```python
from build123d import *
from OCP.BRepFilletAPI import BRepFilletAPI_MakeChamfer

# Parameters (mm, degrees)
BOSS_EXTRUDE1_DEPTH       = 5
FILLET1_R                 = 4
SKETCH2_R                 = 8
BOSS_EXTRUDE2_DEPTH       = 1
SKETCH3_R                 = 8
BOSS_EXTRUDE3_DEPTH       = 1
SKETCH4_R                 = 6
CUT_EXTRUDE1_DEPTH        = 44.235891121
CUT_EXTRUDE2_DEPTH        = 2
CHAMFER1_SIZE             = 1
CHAMFER1_SIZE2            = 1.732050808
CHAMFER1_OF_MIRROR3_SIZE  = 1
CHAMFER1_OF_MIRROR3_SIZE2 = 1.732050808
SKETCH6_R                 = 1.5
CUT_EXTRUDE3_DEPTH        = 42.968348563
CUT_EXTRUDE3_DEPTH_BACK   = 42.968348563


with BuildPart() as part:
    # Sketch1 → Boss-Extrude1 (new, symmetric)
    with BuildSketch(Plane(origin=(0, 0, 0), x_dir=(1, 0, 0), z_dir=(0, 1, 0))):
        with BuildLine():
            Line((-10, 30.489995997), (-10, -2.679491924))
            Line((-10, -2.679491924), (-25.114071484, -6.729295173))
            ThreePointArc((-25.114071484, -6.729295173), (0, -26), (25.114071484, -6.729295173))
            Line((25.114071484, -6.729295173), (10, -2.679491924))
            Line((10, -2.679491924), (10, 30.489995997))
            ThreePointArc((10, 30.489995997), (0, 34), (-10, 30.489995997))
        make_face()
    extrude(amount=BOSS_EXTRUDE1_DEPTH, both=True)

    # Fillet1
    fillet1_edges = [part.edges().sort_by_distance(p)[0] for p in [
        (10, 0, -30.489995997),
        (10, 0, 2.679491924),
        (25.114071484, 0, 6.729295173),
        (-25.114071484, 0, 6.729295173),
        (-10, 0, 2.679491924),
        (-10, 0, -30.489995997),
    ]]
    fillet(fillet1_edges, radius=FILLET1_R)

    # Sketch2 → Boss-Extrude2 (add)
    with BuildSketch(Plane.XZ.offset(5)):
        with Locations(Location((0, 0, 0), (0, 0, 90))):
            Circle(SKETCH2_R)
    extrude(amount=BOSS_EXTRUDE2_DEPTH)

    # Sketch3 → Boss-Extrude3 (add)
    with BuildSketch(Plane(origin=(0, 5, 0), x_dir=(1, 0, 0), z_dir=(0, 1, 0))):
        with Locations(Location((0, 18, 0), (0, 0, 270))):
            Circle(SKETCH3_R)
    extrude(amount=BOSS_EXTRUDE3_DEPTH)

    # Sketch4 → Cut-Extrude1 (cut, through all)
    with BuildSketch(Plane.XZ.offset(6)):
        with Locations(Location((0, 0, 0), (0, 0, 270))):
            Circle(SKETCH4_R)
        with Locations(Location((0, -18, 0), (0, 0, 270))):
            Circle(SKETCH4_R)
    extrude(amount=-CUT_EXTRUDE1_DEPTH, mode=Mode.SUBTRACT)

    # Sketch5 → Cut-Extrude2 (cut)
    with BuildSketch(Plane(origin=(0, 5, 0), x_dir=(1, 0, 0), z_dir=(0, 1, 0))):
        with BuildLine():
            Line((12.188266684, -6.371664756), (20.119713435, -8.496889508))
            ThreePointArc((20.119713435, -8.496889508), (20.768948696, -9.043962883), (20.763662316, -9.892943304))
            ThreePointArc((20.763662316, -9.892943304), (0, -23), (-20.763662316, -9.892943304))
            ThreePointArc((-20.763662316, -9.892943304), (-20.768948696, -9.043962883), (-20.119713435, -8.496889508))
            Line((-20.119713435, -8.496889508), (-12.188266684, -6.371664756))
            ThreePointArc((-12.188266684, -6.371664756), (-11.342355786, -6.086056673), (-10.539679728, -5.695098402))
            ThreePointArc((-10.539679728, -5.695098402), (-9.810114884, -5.592432974), (-9.208235905, -6.017340901))
            ThreePointArc((-9.208235905, -6.017340901), (0, -11), (9.208235905, -6.017340901))
            ThreePointArc((9.208235905, -6.017340901), (9.810114884, -5.592432974), (10.539679728, -5.695098402))
            ThreePointArc((10.539679728, -5.695098402), (11.342355786, -6.086056673), (12.188266684, -6.371664756))
        make_face()
    cut_extrude2 = extrude(amount=-CUT_EXTRUDE2_DEPTH, mode=Mode.SUBTRACT)

    # Chamfer1: one chamfer whose edges measure the first distance from different faces: ONE call of the kernel's chamfer builder (chamfer() names one face for all edges)
    chamfer1_edges_1 = [part.edges().sort_by_distance(p)[0] for p in [
        (9.810114884, 5, 5.592432974),
    ]]
    chamfer1_side_1 = [part.faces().sort_by_distance(p)[0] for p in [
        (9.810114884, 4, 5.592432974),
    ]]
    chamfer1_edges_2 = [part.edges().sort_by_distance(p)[0] for p in [
        (0, 5, 11),
    ]]
    chamfer1_side_2 = [part.faces().sort_by_distance(p)[0] for p in [
        (0, 4, 11),
    ]]
    chamfer1_edges_3 = [part.edges().sort_by_distance(p)[0] for p in [
        (-9.810114884, 5, 5.592432974),
    ]]
    chamfer1_side_3 = [part.faces().sort_by_distance(p)[0] for p in [
        (-9.810114884, 4, 5.592432974),
    ]]
    chamfer1_edges_4 = [part.edges().sort_by_distance(p)[0] for p in [
        (-11.342355786, 5, 6.086056673),
    ]]
    chamfer1_side_4 = [part.faces().sort_by_distance(p)[0] for p in [
        (-11.342355786, 4, 6.086056673),
    ]]
    chamfer1_edges_5 = [part.edges().sort_by_distance(p)[0] for p in [
        (-16.153990059, 5, 7.434277132),
    ]]
    chamfer1_side_5 = [part.faces().sort_by_distance(p)[0] for p in [
        (-16.153990059, 4, 7.434277132),
    ]]
    chamfer1_edges_6 = [part.edges().sort_by_distance(p)[0] for p in [
        (-20.768948696, 5, 9.043962883),
    ]]
    chamfer1_side_6 = [part.faces().sort_by_distance(p)[0] for p in [
        (-20.768948696, 4, 9.043962883),
    ]]
    chamfer1_edges_7 = [part.edges().sort_by_distance(p)[0] for p in [
        (0, 5, 23),
    ]]
    chamfer1_side_7 = [part.faces().sort_by_distance(p)[0] for p in [
        (0, 4, 23),
    ]]
    chamfer1_edges_8 = [part.edges().sort_by_distance(p)[0] for p in [
        (20.768948696, 5, 9.043962883),
    ]]
    chamfer1_side_8 = [part.faces().sort_by_distance(p)[0] for p in [
        (20.768948696, 4, 9.043962883),
    ]]
    chamfer1_edges_9 = [part.edges().sort_by_distance(p)[0] for p in [
        (16.153990059, 5, 7.434277132),
    ]]
    chamfer1_side_9 = [part.faces().sort_by_distance(p)[0] for p in [
        (16.153990059, 4, 7.434277132),
    ]]
    chamfer1_edges_10 = [part.edges().sort_by_distance(p)[0] for p in [
        (11.342355786, 5, 6.086056673),
    ]]
    chamfer1_side_10 = [part.faces().sort_by_distance(p)[0] for p in [
        (11.342355786, 4, 6.086056673),
    ]]
    chamfer1 = BRepFilletAPI_MakeChamfer(part.part.solid().wrapped)
    for e in chamfer1_edges_1:
        chamfer1.Add(CHAMFER1_SIZE, CHAMFER1_SIZE2, e.wrapped, chamfer1_side_1[0].wrapped)  # the first distance lies on this face
    for e in chamfer1_edges_2:
        chamfer1.Add(CHAMFER1_SIZE, CHAMFER1_SIZE2, e.wrapped, chamfer1_side_2[0].wrapped)  # the first distance lies on this face
    for e in chamfer1_edges_3:
        chamfer1.Add(CHAMFER1_SIZE, CHAMFER1_SIZE2, e.wrapped, chamfer1_side_3[0].wrapped)  # the first distance lies on this face
    for e in chamfer1_edges_4:
        chamfer1.Add(CHAMFER1_SIZE, CHAMFER1_SIZE2, e.wrapped, chamfer1_side_4[0].wrapped)  # the first distance lies on this face
    for e in chamfer1_edges_5:
        chamfer1.Add(CHAMFER1_SIZE, CHAMFER1_SIZE2, e.wrapped, chamfer1_side_5[0].wrapped)  # the first distance lies on this face
    for e in chamfer1_edges_6:
        chamfer1.Add(CHAMFER1_SIZE, CHAMFER1_SIZE2, e.wrapped, chamfer1_side_6[0].wrapped)  # the first distance lies on this face
    for e in chamfer1_edges_7:
        chamfer1.Add(CHAMFER1_SIZE, CHAMFER1_SIZE2, e.wrapped, chamfer1_side_7[0].wrapped)  # the first distance lies on this face
    for e in chamfer1_edges_8:
        chamfer1.Add(CHAMFER1_SIZE, CHAMFER1_SIZE2, e.wrapped, chamfer1_side_8[0].wrapped)  # the first distance lies on this face
    for e in chamfer1_edges_9:
        chamfer1.Add(CHAMFER1_SIZE, CHAMFER1_SIZE2, e.wrapped, chamfer1_side_9[0].wrapped)  # the first distance lies on this face
    for e in chamfer1_edges_10:
        chamfer1.Add(CHAMFER1_SIZE, CHAMFER1_SIZE2, e.wrapped, chamfer1_side_10[0].wrapped)  # the first distance lies on this face
    add(Compound.cast(chamfer1.Shape()), mode=Mode.REPLACE)

    # Mirror3: Cut-Extrude2 across plane
    add(cut_extrude2.mirror(Plane.ZX), mode=Mode.SUBTRACT)

    # Chamfer1 of Mirror3: one chamfer whose edges measure the first distance from different faces: ONE call of the kernel's chamfer builder (chamfer() names one face for all edges)
    chamfer1_of_mirror3_edges_1 = [part.edges().sort_by_distance(p)[0] for p in [
        (9.810114884, -5, 5.592432974),
    ]]
    chamfer1_of_mirror3_side_1 = [part.faces().sort_by_distance(p)[0] for p in [
        (9.810114884, -4, 5.592432974),
    ]]
    chamfer1_of_mirror3_edges_2 = [part.edges().sort_by_distance(p)[0] for p in [
        (0, -5, 11),
    ]]
    chamfer1_of_mirror3_side_2 = [part.faces().sort_by_distance(p)[0] for p in [
        (0, -4, 11),
    ]]
    chamfer1_of_mirror3_edges_3 = [part.edges().sort_by_distance(p)[0] for p in [
        (-9.810114884, -5, 5.592432974),
    ]]
    chamfer1_of_mirror3_side_3 = [part.faces().sort_by_distance(p)[0] for p in [
        (-9.810114884, -4, 5.592432974),
    ]]
    chamfer1_of_mirror3_edges_4 = [part.edges().sort_by_distance(p)[0] for p in [
        (-11.342355786, -5, 6.086056673),
    ]]
    chamfer1_of_mirror3_side_4 = [part.faces().sort_by_distance(p)[0] for p in [
        (-11.342355786, -4, 6.086056673),
    ]]
    chamfer1_of_mirror3_edges_5 = [part.edges().sort_by_distance(p)[0] for p in [
        (-16.153990059, -5, 7.434277132),
    ]]
    chamfer1_of_mirror3_side_5 = [part.faces().sort_by_distance(p)[0] for p in [
        (-16.153990059, -4, 7.434277132),
    ]]
    chamfer1_of_mirror3_edges_6 = [part.edges().sort_by_distance(p)[0] for p in [
        (-20.768948696, -5, 9.043962883),
    ]]
    chamfer1_of_mirror3_side_6 = [part.faces().sort_by_distance(p)[0] for p in [
        (-20.768948696, -4, 9.043962883),
    ]]
    chamfer1_of_mirror3_edges_7 = [part.edges().sort_by_distance(p)[0] for p in [
        (0, -5, 23),
    ]]
    chamfer1_of_mirror3_side_7 = [part.faces().sort_by_distance(p)[0] for p in [
        (0, -4, 23),
    ]]
    chamfer1_of_mirror3_edges_8 = [part.edges().sort_by_distance(p)[0] for p in [
        (20.768948696, -5, 9.043962883),
    ]]
    chamfer1_of_mirror3_side_8 = [part.faces().sort_by_distance(p)[0] for p in [
        (20.768948696, -4, 9.043962883),
    ]]
    chamfer1_of_mirror3_edges_9 = [part.edges().sort_by_distance(p)[0] for p in [
        (16.153990059, -5, 7.434277132),
    ]]
    chamfer1_of_mirror3_side_9 = [part.faces().sort_by_distance(p)[0] for p in [
        (16.153990059, -4, 7.434277132),
    ]]
    chamfer1_of_mirror3_edges_10 = [part.edges().sort_by_distance(p)[0] for p in [
        (11.342355786, -5, 6.086056673),
    ]]
    chamfer1_of_mirror3_side_10 = [part.faces().sort_by_distance(p)[0] for p in [
        (11.342355786, -4, 6.086056673),
    ]]
    chamfer1_of_mirror3 = BRepFilletAPI_MakeChamfer(part.part.solid().wrapped)
    for e in chamfer1_of_mirror3_edges_1:
        chamfer1_of_mirror3.Add(CHAMFER1_OF_MIRROR3_SIZE, CHAMFER1_OF_MIRROR3_SIZE2, e.wrapped, chamfer1_of_mirror3_side_1[0].wrapped)  # the first distance lies on this face
    for e in chamfer1_of_mirror3_edges_2:
        chamfer1_of_mirror3.Add(CHAMFER1_OF_MIRROR3_SIZE, CHAMFER1_OF_MIRROR3_SIZE2, e.wrapped, chamfer1_of_mirror3_side_2[0].wrapped)  # the first distance lies on this face
    for e in chamfer1_of_mirror3_edges_3:
        chamfer1_of_mirror3.Add(CHAMFER1_OF_MIRROR3_SIZE, CHAMFER1_OF_MIRROR3_SIZE2, e.wrapped, chamfer1_of_mirror3_side_3[0].wrapped)  # the first distance lies on this face
    for e in chamfer1_of_mirror3_edges_4:
        chamfer1_of_mirror3.Add(CHAMFER1_OF_MIRROR3_SIZE, CHAMFER1_OF_MIRROR3_SIZE2, e.wrapped, chamfer1_of_mirror3_side_4[0].wrapped)  # the first distance lies on this face
    for e in chamfer1_of_mirror3_edges_5:
        chamfer1_of_mirror3.Add(CHAMFER1_OF_MIRROR3_SIZE, CHAMFER1_OF_MIRROR3_SIZE2, e.wrapped, chamfer1_of_mirror3_side_5[0].wrapped)  # the first distance lies on this face
    for e in chamfer1_of_mirror3_edges_6:
        chamfer1_of_mirror3.Add(CHAMFER1_OF_MIRROR3_SIZE, CHAMFER1_OF_MIRROR3_SIZE2, e.wrapped, chamfer1_of_mirror3_side_6[0].wrapped)  # the first distance lies on this face
    for e in chamfer1_of_mirror3_edges_7:
        chamfer1_of_mirror3.Add(CHAMFER1_OF_MIRROR3_SIZE, CHAMFER1_OF_MIRROR3_SIZE2, e.wrapped, chamfer1_of_mirror3_side_7[0].wrapped)  # the first distance lies on this face
    for e in chamfer1_of_mirror3_edges_8:
        chamfer1_of_mirror3.Add(CHAMFER1_OF_MIRROR3_SIZE, CHAMFER1_OF_MIRROR3_SIZE2, e.wrapped, chamfer1_of_mirror3_side_8[0].wrapped)  # the first distance lies on this face
    for e in chamfer1_of_mirror3_edges_9:
        chamfer1_of_mirror3.Add(CHAMFER1_OF_MIRROR3_SIZE, CHAMFER1_OF_MIRROR3_SIZE2, e.wrapped, chamfer1_of_mirror3_side_9[0].wrapped)  # the first distance lies on this face
    for e in chamfer1_of_mirror3_edges_10:
        chamfer1_of_mirror3.Add(CHAMFER1_OF_MIRROR3_SIZE, CHAMFER1_OF_MIRROR3_SIZE2, e.wrapped, chamfer1_of_mirror3_side_10[0].wrapped)  # the first distance lies on this face
    add(Compound.cast(chamfer1_of_mirror3.Shape()), mode=Mode.REPLACE)

    # Sketch6 → Cut-Extrude3 (cut, two sides)
    with BuildSketch(Plane(origin=(0, 0, 0), x_dir=(0, 0, -1), z_dir=(1, 0, 0))) as cut_extrude3_sk:
        Circle(SKETCH6_R)
        with Locations((18, 0)):
            Circle(SKETCH6_R)
    extrude(amount=CUT_EXTRUDE3_DEPTH, mode=Mode.SUBTRACT)
    extrude(cut_extrude3_sk.sketch, amount=-CUT_EXTRUDE3_DEPTH_BACK, mode=Mode.SUBTRACT)


solid = part.part
```
Verification items for the finished model (mm, model axes). A direction names the side the tool comes from. Give positions to 0.01 mm unless a question says otherwise; leave off trailing zeros. Order: outer loops, then holes, each group sorted by start corner. A loop starts at its lowest first (then second) coordinate and runs counter-clockwise, first axis right, second up. Notation, with made-up numbers: M 44.5,-11.75 L 80.5,-11.75 A37 ccw 80.5,25.25 Z; hole C 67,44 d7. An arc over 180 degrees is marked long. Answer in a Markdown table with one row per item. Add a question column.
Item 1: Section check C-C, the plane x = 0. State how many separate pieces and enclosed holes the cut face has, and give its area (3 significant figures).
Item 2: Scan lines: probe 1 along X at (y, z) = (-1.75, -18); probe 2 along Z at (x, y) = (8, 0); probe 3 along Z at (x, y) = (7.95, 0). Record each from-to range of solid material in increasing order. Write a range as from..to.
Item 3: Mould release check, pull along Z, two halves, no side actions. Record for faces 4 (the flat face through (16.986, 0.07, 4.551)), 5 (the cylindrical face through (23.47, 0.07, 7.74)), 6 (the flat face through (0, -3, 14)): released by +Z, released by -Z, zero draft, split by the parting line, or undercut.
Item 4: Section check A-A, the plane y = 0. Enter the section's corners in (x, z).
Item 5: Section check B-B, the plane z = -18. Enter the section's corners in (x, y), and give its area (3 significant figures).
Item 6: Tool access check on faces 1 (the flat face through (16.33, -4.51, 6.57)), 2 (the flat face through (-16.21, 3.51, 7.45)), 3 (the flat face through (-10, 0, -15)). Record the directions out of +Z, -Z, +X, -X, +Y, -Y that give a thin tool (end or side, any length) a straight path to the whole face; none if there is none.
Item 7: Gauge pin test, flat ends, axial feed: pin 1 (10 mm diameter, centred on x = 7.5, z = -5.5, fed in from +Y); pin 2 (3 mm diameter, centred on x = -10, y = 4, fed in from -Z); pin 3 (5 mm diameter, centred on y = 0, z = 0, fed in from +X). Record the tip position at first contact, or that the pin passes through.
Filled sheet:
| question | item | result |
|---|---|---|
| 1 | separate pieces | 3 |
| 1 | enclosed holes | 0 |
| 1 | area | 317 mm^2 |
| 2 | probe 1 | x = -10..-6, 6..10 |
| 2 | probe 2 | z = -31.86..-19.5, -16.5..-1.5, 1.5..24.74 |
| 2 | probe 3 | z = -31.89..-19.5, -16.5..-1.5, 1.5..24.75 |
| 3 | face 4 | released by -Z |
| 3 | face 5 | split by the parting line |
| 3 | face 6 | undercut |
| 4 | outline | M -23.47,11.18 A4 ccw -20.9,5.6 L -12.96,3.47 A4 cw -10.47,1.5 L -5.81,1.5 A6 cw 5.81,1.5 L 10.47,1.5 A4 cw 12.96,3.47 L 20.9,5.6 A4 ccw 23.47,11.18 A26 ccw Z; M -10,-28.39 A4 ccw -8,-31.86 A16 ccw 8,-31.86 A4 ccw 10,-28.39 L 10,-19.5 L 5.81,-19.5 A6 cw -5.81,-19.5 L -10,-19.5 Z; M -10,-16.5 L -5.81,-16.5 A6 cw 5.81,-16.5 L 10,-16.5 L 10,-1.5 L 5.81,-1.5 A6 cw -5.81,-1.5 L -10,-1.5 Z |
| 5 | outline | M -10,-5 L -6,-5 L -6,-1.5 L -10,-1.5 Z; M -10,1.5 L -6,1.5 L -6,6 L -8,6 L -8,5 L -10,5 Z; M 6,-5 L 10,-5 L 10,-1.5 L 6,-1.5 Z; M 6,1.5 L 10,1.5 L 10,5 L 8,5 L 8,6 L 6,6 Z |
| 5 | area | 60.0 mm^2 |
| 6 | face 1 | -Y |
| 6 | face 2 | +Y |
| 6 | face 3 | -Z, -X, +Y, -Y |
| 7 | pin 1 | stops at y = 5 |
| 7 | pin 2 | stops at z = -31.51 |
| 7 | pin 3 | stops at x = 11.23 |
